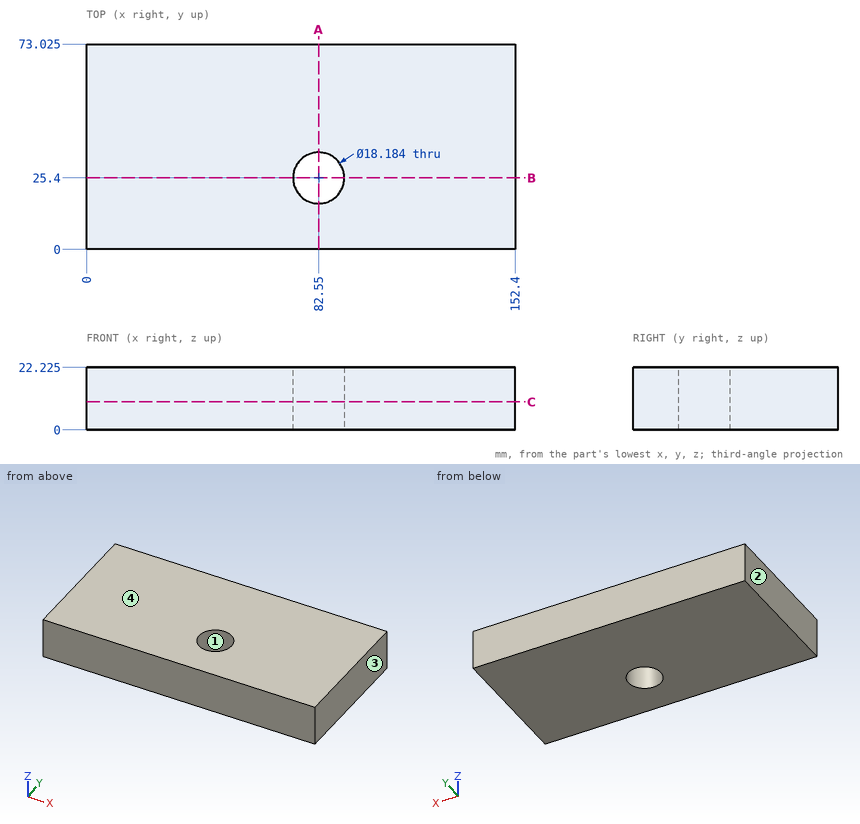
Print and shaded views of the part. All mm, measured from the part's lowest x, y and z. Give positions to 0.01 mm unless a question says otherwise; leave off trailing zeros. Loops run counter-clockwise (first coordinate to the right, second up) from the corner with the lowest first, then second, coordinate; pieces in that order, holes last. Notation, with made-up numbers: (16.25, 1) - (65.25, 1) arc R28 ccw to (65.25, 34) - close; hole circle Ø9 at (-27, 82.25). An arc over 180 degrees is marked (long way). One line per item, written item: value. Start each with the question number.
1. Pull direction X, two halves, no side cores. Call the marked faces 1, 2, 3 and 4: pulls with the +X half, pulls with the -X half, needs draft (parallel to the pull), parting line crosses it, or undercut.
2. Probe L1, parallel to Y at x = 82.55, z = 14.5 (3 decimals); L2, parallel to X at y = 17.5, z = 8; L3, parallel to X at y = 29, z = 4.5. List the from-to ranges inside material, lowest first. Write a range as from..to.
3. Slice it at A-A (x = 82.55). List the corners of the cut face in (y, z) (3 decimals).
4. Slice it at C-C (z = 10). List the corners of the cut face in (x, y) (3 decimals).
5. Slice it at B-B (y = 25.4). List the corners of the cut face in (x, z) (3 decimals).
Solution:
1. face 1: undercut
1. face 2: pulls with the -X half
1. face 3: pulls with the +X half
1. face 4: needs draft
2. L1: y = 0..16.308, 34.492..73.025
2. L2: x = 0..78.05, 87.05..152.4
2. L3: x = 0..74.2, 90.9..152.4
3. outline: (0, 0) - (16.308, 0) - (16.308, 22.225) - (0, 22.225) - close; (34.492, 0) - (73.025, 0) - (73.025, 22.225) - (34.492, 22.225) - close
4. outline: (0, 0) - (152.4, 0) - (152.4, 73.025) - (0, 73.025) - close; hole circle Ø18.184 at (82.55, 25.4)
5. outline: (0, 0) - (73.458, 0) - (73.458, 22.225) - (0, 22.225) - close; (91.642, 0) - (152.4, 0) - (152.4, 22.225) - (91.642, 22.225) - close
